from build123d import *

# Parameters (mm, degrees)
SKETCH1_R           = 4.68
BOSS_EXTRUDE1_DEPTH = 23
SKETCH2_OUTSIDE_W   = 16.668
SKETCH2_OUTSIDE_H   = 16.668
SKETCH2_OUTSIDE_R   = 2.4
CUT_EXTRUDE1_DEPTH  = 20
CHAMFER1_SIZE       = 0.5
CUT_EXTRUDE2_DEPTH  = 2.5
FILLET1_R           = 3.5


with BuildPart() as part:
    # Sketch1 → Boss-Extrude1 (new body)
    with BuildSketch(Plane(origin=(0, 0, 0), x_dir=(1, 0, 0), z_dir=(0, 1, 0))):
        with Locations(Location((0, 0, 0), (0, 0, 270))):
            Circle(SKETCH1_R)
    extrude(amount=BOSS_EXTRUDE1_DEPTH)

    # Sketch2 outside → Cut-Extrude1 (cut)
    with BuildSketch(Plane(origin=(0, 23, 0), x_dir=(1, 0, 0), z_dir=(0, 1, 0))):
        Rectangle(SKETCH2_OUTSIDE_W, SKETCH2_OUTSIDE_H)
        with Locations(Location((0, 0, 0), (0, 0, 270))):
            Circle(SKETCH2_OUTSIDE_R, mode=Mode.SUBTRACT)
    extrude(amount=-CUT_EXTRUDE1_DEPTH, mode=Mode.SUBTRACT)

    # Chamfer1
    chamfer1_edges = [part.edges().sort_by_distance(p)[0] for p in [
        (0, 23, -2.4),
    ]]
    chamfer(chamfer1_edges, length=CHAMFER1_SIZE)

    # Sketch8 → Cut-Extrude2 (cut)
    with BuildSketch(Plane.XZ):
        Polygon((1.870614872, 0), (0.935307436, 1.62), (-0.935307436, 1.62), (-1.870614872, 0), (-0.935307436, -1.62), (0.935307436, -1.62), align=None)
    extrude(amount=-CUT_EXTRUDE2_DEPTH, mode=Mode.SUBTRACT)

    # Fillet1
    # the kernel refuses this fillet: 3.5 mm, written as the material it takes off along each edge
    with BuildSketch(Plane(origin=(0, 0, 0), x_dir=(0, 0, 1), z_dir=(-1, 0, 0))) as fillet1_piece_1:
        with BuildLine():
            CenterArc((1.215898385, 3.5), FILLET1_R, 270, 81.786789298)
            Line((1.215898385, 0), (1.215898385, -0.07))
            Line((1.215898385, -0.07), (4.68, -0.07))
            Line((4.68, -0.07), (4.75, 0))
            ThreePointArc((4.75, 0), (4.75, 1.5), (4.749282032, 2.99))
            Line((4.749282032, 2.99), (4.68, 3))
        make_face()
    revolve(axis=Axis((0, 0, 0), (0, 1, 0)), mode=Mode.SUBTRACT)


solid = part.part
Could you check a few things on this model? Use its own coordinates, in mm. A direction names the side the tool comes from. Coordinates: 2 decimals unless noted, no trailing zeros. Loops run counter-clockwise (first coordinate to the right, second up) from the corner with the lowest first, then second, coordinate; pieces in that order, holes last.
1. I need wall thicknesses on L1, parallel to X at y = 1.75, z = -0.5; L2, parallel to Y at x = -2.75, z = 1.75; L3, parallel to X at y = 13, z = 0.25. Which ranges of each line are inside material? Lowest first, please.
2. For faces 5 (the face through (2, 3, 2)), 6 (the face through (0, 1, -1.62)), which set-ups out of +Z, -Z, +X, -X, +Y, -Y let a thin tool reach every point of the face, with its end or its side?
3. For P1, Ø2, axis at x = 3.5, z = -2.5, coming from the +Y side; P2, Ø4, axis at x = -1, y = 14, coming from the +Z side; P3, Ø2, axis at x = 2.5, z = -3, coming from the -Y side, each with a flat end and sliding along its axis, tell me the tip position at first contact or that it passes through.
4. We'd pull the mould along Z, two halves only. Please class faces 1 (the face through (1.41, 1.24, 0.8)), 2 (the face through (-1.396, 1.244, 0.821)), 3 (the face through (0, 23, 0)), 4 (the face through (2.024, 12.886, 1.29)): released by +Z, released by -Z, zero draft, split by the parting line, or undercut.
5. Imagine slicing it at A-A (y = 7.75). Please give me the cut outline in (x, z).
Computed values:
1. L1: x = -4.22 to -1.58, 1.58 to 4.22
1. L2: y = 0.66 to 3
1. L3: x = -2.39 to 2.39
2. face 5: +Y
2. face 6: -Y
3. P1: stops at y = 3
3. P2: stops at z = 2.4
3. P3: stops at y = 0.43
4. face 1: undercut
4. face 2: undercut
4. face 3: zero draft
4. face 4: split by the parting line
5. outline: circle Ø4.8 at (0, 0)
